Design review of the part built by this model. Coordinates are the model's own, in mm. Face numbers are marked on the shaded views. A direction names the side the tool comes from. Give positions to 0.01 mm unless a question says otherwise; leave off trailing zeros. Order: outer loops, then holes, each group sorted by start corner. A loop starts at its lowest first (then second) coordinate and runs counter-clockwise, first axis right, second up. Notation, with made-up numbers: (66, 45) -> (92, 45) arc R17 ccw to (92, 53) -> close; hole circle Ø7 at (84.5, 64.25). An arc over 180 degrees is marked (long way). Return JSON: item names as keys, results as strings.
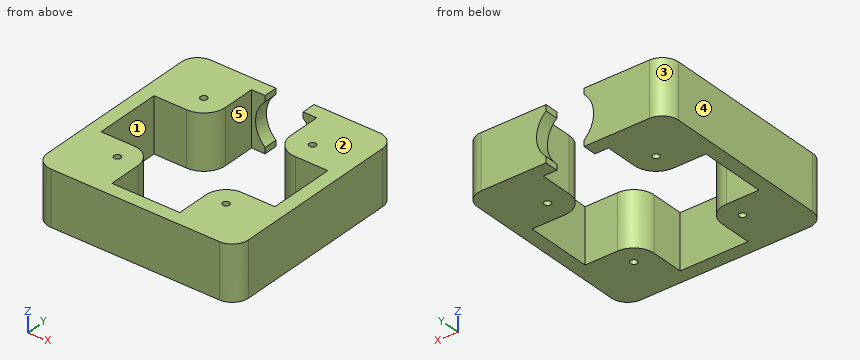
```python
from build123d import *

# Parameters (mm, degrees)
F1_DEPTH = 20
F3_DEPTH = 25
F6_D     = 2.5


with BuildPart() as f1:
    # F0 (on Top) → F1 (new body)
    with BuildSketch(Plane.XY):
        with BuildLine():
            Line((0, 68), (0, 6))
            ThreePointArc((0, 6), (1.757359, 1.757359), (6, 0))
            Line((6, 0), (37, 0))
            Line((37, 0), (68, 0))
            ThreePointArc((68, 0), (72.242641, 1.757359), (74, 6))
            Line((74, 6), (74, 68))
            ThreePointArc((74, 68), (72.242641, 72.242641), (68, 74))
            Line((68, 74), (44, 74))
            Line((44, 74), (44, 69))
            Line((44, 69), (49, 69))
            Line((49, 69), (49, 57))
            ThreePointArc((49, 57), (51.343146, 51.343146), (57, 49))
            Line((57, 49), (69, 49))
            Line((69, 49), (69, 24.5))
            Line((69, 24.5), (57, 24.5))
            ThreePointArc((57, 24.5), (51.696699, 22.303301), (49.5, 17))
            Line((49.5, 17), (49.5, 5))
            Line((49.5, 5), (24.5, 5))
            Line((24.5, 5), (24.5, 17))
            ThreePointArc((24.5, 17), (22.303301, 22.303301), (17, 24.5))
            Line((17, 24.5), (5, 24.5))
            Line((5, 24.5), (5, 49))
            Line((5, 49), (17, 49))
            ThreePointArc((17, 49), (22.656854, 51.343146), (25, 57))
            Line((25, 57), (25, 69))
            Line((25, 69), (30, 69))
            Line((30, 69), (30, 74))
            Line((30, 74), (6, 74))
            ThreePointArc((6, 74), (1.757359, 72.242641), (0, 68))
        make_face()
    extrude(amount=F1_DEPTH)


with BuildPart() as f3:
    # F2 (on face) → F3 (new body)
    with BuildSketch(Plane(origin=(0, 74, 0), x_dir=(-1, 0, 0), z_dir=(0, 1, 0))):
        with BuildLine():
            ThreePointArc((-26.5, 10), (-37, 20.5), (-47.5, 10))
            Line((-47.5, 10), (-26.5, 10))
        make_face()
        with BuildLine():
            Line((-26.5, 10), (-47.5, 10))
            ThreePointArc((-47.5, 10), (-37, -0.5), (-26.5, 10))
        make_face()
    extrude(amount=-F3_DEPTH)


with BuildPart() as f1_1:
    add(f1.part)

    # F4: cut F3
    add(f3.part, mode=Mode.SUBTRACT)

    # F6 (through all)
    with Locations(Plane.XY.offset(20)):
        with Locations((17, 57), (57, 57), (57, 17), (17, 17)):
            Hole(F6_D / 2)


solid = f1_1.part
```
Item 1: Machinability: for the marked faces 4 and 5, which of the approach directions +Z, -Z, +X, -X, +Y, -Y give a long, thin tool a straight path to every point of the face, cutting with its end or side? Answer none if there is none.
Result set:
{"face 4": "+Z, -Z, -X, +Y, -Y", "face 5": "+Z, -Z"}
Item 2: Add section A-A (y = 35). Give the boundary of the cut face in (x, z), plus the area to 3 significant figures.
Result set:
{"outline": "(0, 0) -> (5, 0) -> (5, 20) -> (0, 20) -> close; (69, 0) -> (74, 0) -> (74, 20) -> (69, 20) -> close", "area": "200 mm^2"}
Item 3: For pin 1 (2 mm diameter, centred on x = 57, y = 17, fed in from +Z); pin 2 (2.5 mm diameter, centred on y = 71, z = 19, fed in from +X); pin 3 (1.7 mm diameter, centred on y = 70.5, z = 1.5, fed in from +X), all flat-tipped, find the tip position at first contact; note any pin that passes through.
Result set:
{"pin 1": "passes through", "pin 2": "stops at x = 73.74", "pin 3": "stops at x = 73.77"}
Item 4: Add section B-B (x = 10.5). Give the boundary of the cut face in (y, z).
Result set:
{"outline": "(0, 0) -> (24.5, 0) -> (24.5, 20) -> (0, 20) -> close; (49, 0) -> (74, 0) -> (74, 20) -> (49, 20) -> close"}
Item 5: Wall thickness on L1, parallel to Y at x = 17, z = 5; L2, parallel to X at y = 67, z = 1; L3, parallel to X at y = 8, z = 1: over which ranges is each line inside the solid? List them lowest first. Write a range as [from, to].
Result set:
{"L1": "y = [0, 15.75], [18.25, 24.5], [49, 55.75], [58.25, 74]", "L2": "x = [0, 25], [49, 74]", "L3": "x = [0, 24.5], [49.5, 74]"}
Item 6: Add section C-C (z = 4.75). Give the number of separate pieces and of enclosed holes in the cut face, plus the area to 3 significant figures.
Result set:
{"separate pieces": "1", "enclosed holes": "4", "area": "2,750 mm^2"}
Item 7: Mouldability with a two-part tool opening along Y and no side actions: class the marked faces 1, 2 and 3 as released by +Y, released by -Y, zero draft, split by the parting line, or undercut.
Result set:
{"face 1": "undercut", "face 2": "zero draft", "face 3": "released by +Y"}
